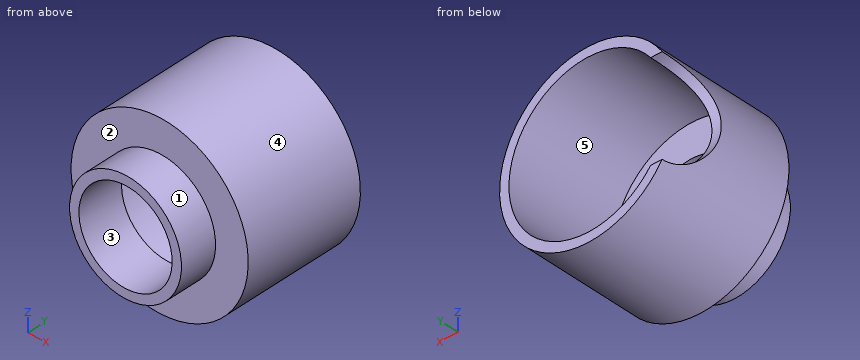
from build123d import *

# Parameters (mm, degrees)
SKETCH3_R          = 10.45
CUT_EXTRUDE1_DEPTH = 44.571665105


with BuildPart() as part:
    # Sketch2 → Revolve1 (revolve)
    with BuildSketch(Plane.XY, mode=Mode.PRIVATE) as revolve1_sk:
        Polygon((10, 0), (10, 10), (17, 10), (17, 34.3), (19, 34.3), (19, 8), (12, 8), (12, 0), align=None)
    revolve(revolve1_sk.sketch.rotate(Axis((0, 0, 0), (0, 1, 0)), 90), axis=Axis((0, 0, 0), (0, 1, 0)))

    # Sketch3 → Cut-Extrude1 (cut, through all)
    with BuildSketch(Plane(origin=(0, 0, 0), x_dir=(0, 0, -1), z_dir=(1, 0, 0))):
        with Locations((0, 34.3)):
            Circle(SKETCH3_R)
    extrude(amount=-CUT_EXTRUDE1_DEPTH, mode=Mode.SUBTRACT)


solid = part.part
Could you check a few things on this model? Use its own coordinates, in mm. Face numbers are marked on the shaded views. A direction names the side the tool comes from. Coordinates: 2 decimals unless noted, no trailing zeros. Write each loop counter-clockwise with the first axis right and the second up, starting at its lowest first coordinate (ties: lowest second). Pieces come first, ordered by that corner, then holes. Notation, with made-up numbers: (-40, 73.5) - (-15, 73.5) arc R28 cw to (-15, 109.5) - close; hole circle Ø5 at (48, 89.5). An arc over 180 degrees is marked (long way). Put each result on its own line as item: value. Start each with the question number.
Q1. Which directions (+Z, -Z, +X, -X, +Y, -Y) give clear straight access to the entire face, cutting with the end or side of a thin tool? Please do the marked faces 4 and 5.
Q2. I want a section at B-B on z = 6.5. Write out the boundary of the cut face in (x, y), plus the area to 3 significant figures.
Q3. Thinking about a two-plate mould opening in X: for the marked faces 1, 2 and 3, which applies, pulls with the +X half, pulls with the -X half, needs draft (parallel to the pull), parting line crosses it, or undercut?
Q4. I want a section at D-D on x = 11. Write out the boundary of the cut face in (y, z), plus the area to 3 significant figures.
Q5. I'm going to push flat-ended pins straight in: P1, Ø12, axis at x = 3, z = -6.5, coming from the +Y side; P2, Ø8, axis at x = 5.5, y = 16, coming from the -Z side; P3, Ø2, axis at y = 25, z = -6, coming from the -X side. Where does each tip first touch, or does it pass through?
Q6. I want a section at A-A on x = 0. Write out the boundary of the cut face in (y, z).
Q7. I want a section at C-C on y = 5.5. Write out the boundary of the cut face in (x, z), plus the area to 3 significant figures.
Q8. Please list where these lines run through material, in increasing order: L1, parallel to X at y = 20, z = 0; L2, parallel to X at y = 6, z = 0; L3, parallel to Y at x = -15, z = 11.
Checks:
1. face 4: +Y, -Y
1. face 5: +Y
2. outline: (-17.85, 8) - (-10.09, 8) - (-10.09, 0) - (-7.6, 0) - (-7.6, 10) - (-15.71, 10) - (-15.71, 26.12) - (-17.85, 26.12) - close; (7.6, 0) - (10.09, 0) - (10.09, 8) - (17.85, 8) - (17.85, 34.3) - (15.71, 34.3) - (15.71, 10) - (7.6, 10) - close
2. area: 168 mm²
3. face 1: parting line crosses it
3. face 2: needs draft
3. face 3: undercut
4. outline: (0, -4.8) - (8, -4.8) - (8, -15.49) - (34.3, -15.49) - (34.3, -12.96) - (10, -12.96) - (10, 12.96) - (34.3, 12.96) - (34.3, 15.49) - (8, 15.49) - (8, 4.8) - (0, 4.8) - close
4. area: 262 mm²
5. P1: y = 10
5. P2: z = -18.94
5. P3: x = -18.33
6. outline: (0, -12) - (8, -12) - (8, -19) - (34.3, -19) - (34.3, -17) - (10, -17) - (10, -10) - (0, -10) - close; (0, 10) - (10, 10) - (10, 17) - (34.3, 17) - (34.3, 19) - (8, 19) - (8, 12) - (0, 12) - close
7. outline: circle Ø24 at (0, 0); hole circle Ø20 at (0, 0)
7. area: 138 mm²
8. L1: -19 to -17, 17 to 19
8. L2: -12 to -10, 10 to 12
8. L3: 8 to 34.3
